```python
from build123d import *

# Parameters (mm, degrees)
F0_W     = 235
F0_H     = 110
F2_T     = -1
F4_DEPTH = 1


with BuildPart() as f1:
    # F0 (on Front) → F1 (revolve)
    with BuildSketch(Plane.XZ):
        with Locations((-117.5, 55)):
            Rectangle(F0_W, F0_H)
    revolve(axis=Axis((0, 0, 55), (0, 0, -1)))

    # F2
    f2_openings = [f1.faces().sort_by_distance(p)[0] for p in [
        (0, 0, 0),
    ]]
    offset(amount=F2_T, openings=f2_openings)


with BuildPart() as f4:
    # F3 (on face) → F4 (new body)
    with BuildSketch(Plane.XY.offset(110)):
        with BuildLine():
            ThreePointArc((235, 0), (166.170094, 166.170094), (0, 235))
            ThreePointArc((0, 235), (-166.170094, -166.170094), (235, 0))
        make_face()
        with BuildLine():
            ThreePointArc((140, 55), (-98.994949, -43.994949), (0, 195))
            ThreePointArc((0, 195), (98.994949, 153.994949), (140, 55))
        make_face(mode=Mode.SUBTRACT)
        with BuildLine():
            ThreePointArc((140, 55), (98.994949, 153.994949), (0, 195))
            ThreePointArc((0, 195), (-98.994949, -43.994949), (140, 55))
        make_face()
        with BuildLine():
            ThreePointArc((75, 55), (-53.033009, 1.966991), (0, 130))
            ThreePointArc((0, 130), (53.033009, 108.033009), (75, 55))
        make_face(mode=Mode.SUBTRACT)
    extrude(amount=F4_DEPTH)


solid = f4.part
```
Could you check a few things on this model? Use its own coordinates, in mm. Round coordinates to 2 decimals unless told otherwise and drop trailing zeros. Loops run counter-clockwise (first coordinate to the right, second up) from the corner with the lowest first, then second, coordinate; pieces in that order, holes last. Notation, with made-up numbers: M 43,17 L 100,17 A33 ccw 100,56 Z; hole C -33,-19.75 d5. An arc over 180 degrees is marked long. Put each result on its own line as item: value.
Q1. Imagine slicing it at C-C (z = 110.5). Write out the boundary of the cut face in (x, y).
Check result:
outline: M 0,235 A235 ccw long 235,0 A235 ccw Z; hole M 0,130 A75 ccw long 75,55 A75 ccw Z
Q2. Imagine slicing it at D-D (x = -172.5). Write out the boundary of the cut face in (y, z).
Check result:
outline: M -159.59,110 L 159.59,110 L 159.59,111 L -159.59,111 Z
Q3. Imagine slicing it at A-A (y = 88.5). Write out the boundary of the cut face in (x, z).
Check result:
outline: M -217.7,110 L -67.1,110 L -67.1,111 L -217.7,111 Z; M 67.1,110 L 217.7,110 L 217.7,111 L 67.1,111 Z
Q4. Imagine slicing it at B-B (x = -19). Write out the boundary of the cut face in (y, z).
Check result:
outline: M -234.23,110 L -17.55,110 L -17.55,111 L -234.23,111 Z; M 127.55,110 L 234.23,110 L 234.23,111 L 127.55,111 Z
Q5. I need wall thicknesses on probe 1 along X at (y, z) = (72, 110.75); probe 2 along Y at (x, z) = (-59, 110.4); probe 3 along Y at (x, z) = (10, 110.55). Which ranges of each line are inside material? Lowest first, please.
Check result:
probe 1: -223.7 to -73.05, 73.05 to 223.7
probe 2: -227.47 to 8.7, 101.3 to 227.47
probe 3: -234.79 to -19.33, 129.33 to 234.79
